Source: CAD feature listing. Evaluate the final solid. Frame: model axes, mm. A direction names the side the tool comes from. Round coordinates to 2 decimals unless told otherwise and drop trailing zeros. Write each loop counter-clockwise with the first axis right and the second up, starting at its lowest first coordinate (ties: lowest second). Pieces come first, ordered by that corner, then holes. Notation, with made-up numbers: (7, 2) -> (63, 2) arc R10 cw to (63, 19) -> close; hole circle Ø3 at (13.5, 43.5). An arc over 180 degrees is marked (long way). Return JSON: item names as keys, results as strings. Group by question number.
from build123d import *

# Parameters (mm, degrees)
PROFILE_SHAPE_DEPTH            = 5
SKETCH2_R                      = 4
LOWER_HOLE_DEPTH               = 11
SKETCH3_R                      = 4
UPPER_HOLE_RIGHT_DEPTH         = 11
M6_TAPPED_HOLE_TOP_D           = 5
M6_TAPPED_HOLE_TOP_DEPTH       = 15
M6_TAPPED_HOLE_TOP_CSINK_D     = 6.05
M6_TAPPED_HOLE_TOP_CSINK_ANGLE = 90
M6_TAPPED_HOLE_TOP_TIP         = 1.502151548
EXTERNAL_EDGES_SIZE            = 2
INTERNAL_EDGES_R               = 5


with BuildPart() as part:
    # Sketch1 → Profile Shape (new body, symmetric)
    with BuildSketch(Plane.XY):
        Polygon((-10, -10), (-10, 40), (-40, 40), (-40, 60), (40, 60), (40, 40), (10, 40), (10, -10), align=None)
    extrude(amount=PROFILE_SHAPE_DEPTH, both=True)

    # Sketch2 → Lower Hole (cut, through all)
    with BuildSketch(Plane.XY.offset(5)):
        Circle(SKETCH2_R)
    extrude(amount=-LOWER_HOLE_DEPTH, mode=Mode.SUBTRACT)

    # Sketch3 → Upper Hole Right (cut, through all)
    with BuildSketch(Plane.XY.offset(5)):
        with Locations((26.9, 50)):
            Circle(SKETCH3_R)
    upper_hole_right = extrude(amount=-UPPER_HOLE_RIGHT_DEPTH, mode=Mode.SUBTRACT)

    # Upper Hole Left: Upper Hole Right across plane
    add(upper_hole_right.mirror(Plane(origin=(0, 0, 0), x_dir=(0, 0, 1), z_dir=(1, 0, 0))), mode=Mode.SUBTRACT)

    # M6 Tapped Hole Top
    with Locations(Plane(origin=(0, 60, 0), x_dir=(1, 0, 0), z_dir=(0, 1, 0))):
        with Locations((0, 0)):
            CounterSinkHole(M6_TAPPED_HOLE_TOP_D / 2, M6_TAPPED_HOLE_TOP_CSINK_D / 2, depth=M6_TAPPED_HOLE_TOP_DEPTH, counter_sink_angle=M6_TAPPED_HOLE_TOP_CSINK_ANGLE)
            with Locations((0, 0, -(M6_TAPPED_HOLE_TOP_DEPTH + M6_TAPPED_HOLE_TOP_TIP / 2))):  # 118° drill point
                Cone(0, M6_TAPPED_HOLE_TOP_D / 2, M6_TAPPED_HOLE_TOP_TIP, mode=Mode.SUBTRACT)

    # External Edges
    external_edges_edges = [part.edges().sort_by_distance(p)[0] for p in [
        (-10, -10, 0),
        (-40, 40, 0),
        (-40, 60, 0),
        (40, 60, 0),
        (40, 40, 0),
        (10, -10, 0),
    ]]
    chamfer(external_edges_edges, length=EXTERNAL_EDGES_SIZE)

    # Internal Edges
    internal_edges_edges = [part.edges().sort_by_distance(p)[0] for p in [
        (-10, 40, 0),
        (10, 40, 0),
    ]]
    fillet(internal_edges_edges, radius=INTERNAL_EDGES_R)


solid = part.part
Item 1: Pull-direction query (Z, two-part tool) for faces 1 (the flat face through (1, 33, 5)), 2 (the conical face through (-0.094, 43.759, 0.424)), 3 (the flat face through (10, 14, 0)), 4 (the flat face through (1, 33, -5)); classes: +Z half, -Z half, draft (parallel to the pull), parting line (faces both ways), or undercut.
Item 2: First-contact query: pin 1 Ø13 at (x, y) = (0, 0) entering from +Z; pin 2 Ø3 at (y, z) = (28.5, 3.5) entering from -X; pin 3 Ø3 at (y, z) = (38, 0.5) entering from -X; pin 4 Ø3 at (x, z) = (-32, -2.5) entering from -Y. Flat tips, straight axial feed; report the tip coordinate or a pass-through.
Item 3: Cut plane A-A on x = -26.9. Output: boundary loops of the cut face in (y, z).
Item 4: Cut plane D-D on z = -1.5. Give the number of separate pieces and of enclosed holes in the cut face, and give its area (3 significant figures).
Item 5: Cut plane C-C on x = 22. Output: boundary loops of the cut face in (y, z), and give its area (3 significant figures).
Item 6: Set-up query: faces 5 (the flat face through (27, 40, 0)), 6 (the flat face through (-26, 40, 0)), 7 (the flat face through (-0.5, 60, 3.4)). Return all of +Z, -Z, +X, -X, +Y, -Y with unobstructed straight access to the full face (end or side cutting, diameter ignored); none if empty.
Item 7: Material intervals for probe 1 along Y at (x, z) = (-26.9, -0.5); probe 2 along Z at (x, y) = (0, 50); probe 3 along X at (y, z) = (28, 4), sorted ascending.
Item 8: Cut plane B-B on y = 0. Output: boundary loops of the cut face in (x, z), and give its area (3 significant figures).
Here are the results:
{
 "1": {"face 1": "+Z half", "face 2": "undercut", "face 3": "draft", "face 4": "-Z half"},
 "2": {"pin 1": "stops at z = 5", "pin 2": "stops at x = -10", "pin 3": "stops at x = -12.82", "pin 4": "stops at y = 40"},
 "3": {"outline": "(40, -5) -> (46, -5) -> (46, 5) -> (40, 5) -> close; (54, -5) -> (60, -5) -> (60, 5) -> (54, 5) -> close"},
 "4": {"separate pieces": "1", "enclosed holes": "3", "area": "2,390 mm^2"},
 "5": {"outline": "(40, -5) -> (60, -5) -> (60, 5) -> (40, 5) -> close", "area": "200 mm^2"},
 "6": {"face 5": "+Z, -Z, +X, -Y", "face 6": "+Z, -Z, -X, -Y", "face 7": "+Z, -Z, +X, -X, +Y"},
 "7": {"probe 1": "y = 40 to 46, 54 to 60", "probe 2": "z = -5 to -2.5, 2.5 to 5", "probe 3": "x = -10 to 10"},
 "8": {"outline": "(-10, -5) -> (-4, -5) -> (-4, 5) -> (-10, 5) -> close; (4, -5) -> (10, -5) -> (10, 5) -> (4, 5) -> close", "area": "120 mm^2"}
}
